```python
from build123d import *

# Parameters (mm, degrees)
BOSS_EXTRUDE2_DEPTH = 3
CUT_EXTRUDE1_REACH  = 5


with BuildPart() as part:
    # Sketch1 → Boss-Extrude2 (new body)
    with BuildSketch(Plane.XY):
        with BuildLine():
            Line((-19.985447982, 0.762803358), (-59.956343946, 2.288410074))
            ThreePointArc((-59.956343946, 2.288410074), (-55.730717245, 22.228071336), (-45.073672701, 39.602576043))
            Line((-45.073672701, 39.602576043), (-13.592462366, 14.67122922))
            ThreePointArc((-13.592462366, 14.67122922), (-18.172234131, 8.352838241), (-19.985447982, 0.762803358))
        make_face()
    extrude(amount=BOSS_EXTRUDE2_DEPTH)

    # Sketch2 → Cut-Extrude1 (cut, up to next)
    with BuildSketch(Plane.XY.offset(3), mode=Mode.PRIVATE) as cut_extrude1_sk1:
        with BuildLine():
            Line((-45.58858723, 35.856390146), (-17.292222743, 13.600699711))
            ThreePointArc((-17.292222743, 13.600699711), (-17.980329977, 12.677055412), (-18.619154377, 11.718664185))
            Line((-18.619154377, 11.718664185), (-49.08686154, 30.894660124))
            ThreePointArc((-49.08686154, 30.894660124), (-47.402688122, 33.421327903), (-45.58858723, 35.856390146))
        make_face()
    cut_extrude1_tool1 = extrude(cut_extrude1_sk1.sketch, amount=-CUT_EXTRUDE1_REACH, mode=Mode.PRIVATE) & part.part
    add(cut_extrude1_tool1.solids().sort_by_distance((-34.882242, 24.593771, 3))[0], mode=Mode.SUBTRACT)
    # Sketch2 → Cut-Extrude1 (cut, up to next)
    with BuildSketch(Plane.XY.offset(3), mode=Mode.PRIVATE) as cut_extrude1_sk2:
        with BuildLine():
            Line((-52.047329922, 25.59444174), (-19.74209066, 9.708236522))
            ThreePointArc((-19.74209066, 9.708236522), (-20.223124653, 8.661710528), (-20.648728467, 7.591443388))
            Line((-20.648728467, 7.591443388), (-54.437556866, 20.013805296))
            ThreePointArc((-54.437556866, 20.013805296), (-53.315510448, 22.835418665), (-52.047329922, 25.59444174))
        make_face()
    cut_extrude1_tool2 = extrude(cut_extrude1_sk2.sketch, amount=-CUT_EXTRUDE1_REACH, mode=Mode.PRIVATE) & part.part
    add(cut_extrude1_tool2.solids().sort_by_distance((-39.233314, 16.803912, 3))[0], mode=Mode.SUBTRACT)
    # Sketch2 → Cut-Extrude1 (cut, up to next)
    with BuildSketch(Plane.XY.offset(3), mode=Mode.PRIVATE) as cut_extrude1_sk3:
        with BuildLine():
            Line((-56.231354546, 14.213893413), (-21.329134483, 5.391476812))
            ThreePointArc((-21.329134483, 5.391476812), (-21.58207174, 4.267807331), (-21.775854038, 3.132440087))
            Line((-21.775854038, 3.132440087), (-57.409069737, 8.25825114))
            ThreePointArc((-57.409069737, 8.25825114), (-56.898189132, 11.251492055), (-56.231354546, 14.213893413))
        make_face()
    cut_extrude1_tool3 = extrude(cut_extrude1_sk3.sketch, amount=-CUT_EXTRUDE1_REACH, mode=Mode.PRIVATE) & part.part
    add(cut_extrude1_tool3.solids().sort_by_distance((-41.869702, 8.279642, 3))[0], mode=Mode.SUBTRACT)


solid = part.part
```
Input: part model. Units: mm. Frame: model coordinates. A direction names the side the tool comes from. Coordinates: 2 decimals unless noted, no trailing zeros. Loops run counter-clockwise (first coordinate to the right, second up) from the corner with the lowest first, then second, coordinate; pieces in that order, holes last. Notation, with made-up numbers: (7, 12) -> (47, 12) arc R7 ccw to (47, 16) -> close; hole circle Ø4 at (-40, 66). An arc over 180 degrees is marked (long way). Use a Markdown table: item, result.
1) Access query for faces 1 (the cylindrical face through (-56.906, 11.21, 1.521)), 2 (the flat face through (-39.691, 1.515, 1.479)). Directions: +Z, -Z, +X, -X, +Y, -Y. A direction counts if a zero-diameter tool reaches every point of the face in a straight line with its end or side. Return the directions, or none.
Results found:
| item | result |
|---|---|
| face 1 | +Z, -Z |
| face 2 | +Z, -Z, -X, -Y |
2) Material intervals for line 1 along Y through (x, z) = (-47, 2.65); line 2 along Y through (x, z) = (-23.5, 0.4); line 3 along X through (y, z) = (23.5, 2.1), sorted ascending. Write a range as from..to.
Results found:
| item | result |
|---|---|
| line 1 | y = 1.79..6.76, 11.88..17.28, 23.11..29.58, 33.99..37.3 |
| line 2 | y = 0.9..3.38, 5.94..8.64, 11.56..14.79, 18.48..22.52 |
| line 3 | x = -55.21..-53.03, -47.79..-37.34, -29.88..-24.74 |
3) Contact query for a flat-ended pin moving along its axis: pin 1 (1 mm diameter, centred on x = -34.5, y = 25, fed in from +Z). Output: stop coordinate, or through.
Results found:
| item | result |
|---|---|
| pin 1 | passes through |
4) Cut plane C-C (z = 1.3). Return the cut outline in (x, y), then the cut area to 3 significant figures.
Results found:
| item | result |
|---|---|
| outline | (-59.96, 2.29) -> (-19.99, 0.76) arc R20 cw to (-13.59, 14.67) -> (-45.07, 39.6) arc R60 ccw to start; hole (-57.41, 8.26) -> (-21.78, 3.13) arc R22 cw to (-21.33, 5.39) -> (-56.23, 14.21) arc R58 ccw to start; hole (-54.44, 20.01) -> (-20.65, 7.59) arc R22 cw to (-19.74, 9.71) -> (-52.05, 25.59) arc R58 ccw to start; hole (-49.09, 30.89) -> (-18.62, 11.72) arc R22 cw to (-17.29, 13.6) -> (-45.59, 35.86) arc R58 ccw to start |
| area | 681 mm2 |
5) Pull-direction query (Y, two-part tool) for faces 3 (the cylindrical face through (-18.126, 8.453, 1.479)), 4 (the cylindrical face through (-17.97, 12.69, 1.52)), 5 (the cylindrical face through (-55.836, 21.961, 1.479)); classes: released by +Y, released by -Y, zero draft, split by the parting line, or undercut.
Results found:
| item | result |
|---|---|
| face 3 | released by -Y |
| face 4 | undercut |
| face 5 | released by +Y |
6) Cut plane D-D (y = 34). Return the cut outline in (x, z), then the cut area to 3 significant figures.
Results found:
| item | result |
|---|---|
| outline | (-49.44, 0) -> (-46.99, 0) -> (-46.99, 3) -> (-49.44, 3) -> close; (-43.23, 0) -> (-38, 0) -> (-38, 3) -> (-43.23, 3) -> close |
| area | 23.0 mm2 |
7) Cut plane B-B (y = 24). Return the cut outline in (x, z).
Results found:
| item | result |
|---|---|
| outline | (-54.99, 0) -> (-52.8, 0) -> (-52.8, 3) -> (-54.99, 3) -> close; (-48.8, 0) -> (-38.13, 0) -> (-38.13, 3) -> (-48.8, 3) -> close; (-30.51, 0) -> (-25.37, 0) -> (-25.37, 3) -> (-30.51, 3) -> close |
8) Cut plane A-A (x = -29). Return the cut outline in (y, z).
Results found:
| item | result |
|---|---|
| outline | (1.11, 0) -> (4.17, 0) -> (4.17, 3) -> (1.11, 3) -> close; (7.33, 0) -> (10.66, 0) -> (10.66, 3) -> (7.33, 3) -> close; (14.26, 0) -> (18.25, 0) -> (18.25, 3) -> (14.26, 3) -> close; (22.81, 0) -> (26.87, 0) -> (26.87, 3) -> (22.81, 3) -> close |
